from build123d import *

# Parameters (mm, degrees)
SKETCH_1_W          = 22
SKETCH_1_H          = 22
EXTRUDE_1_DEPTH     = 12
SKETCH_3_R          = 3.5
CUT_EXTRUDE_2_DEPTH = 12
SKETCH_5_R          = 1.5
EXTRUDE_2_DEPTH     = 4
SKETCH_6_W          = 12
SKETCH_6_H          = 22
EXTRUDE_3_DEPTH     = 22
SKETCH_7_R          = 4
CUT_EXTRUDE_3_DEPTH = 22


with BuildPart() as part:
    # 草图1 → 凸台-拉伸1 (new body)
    with BuildSketch(Plane.XY):
        Rectangle(SKETCH_1_W, SKETCH_1_H)
    extrude(amount=EXTRUDE_1_DEPTH)

    # 草图3 → 切除-拉伸2 (cut)
    with BuildSketch(Plane.XY.offset(12)):
        Circle(SKETCH_3_R)
    extrude(amount=-CUT_EXTRUDE_2_DEPTH, mode=Mode.SUBTRACT)

    # 草图5 → 凸台-拉伸2 (add)
    with BuildSketch(Plane(origin=(0, 0, 0), x_dir=(-1, 0, 0), z_dir=(0, 0, -1))):
        with Locations(Location((0, 8, 0), (0, 0, 180))):
            Circle(SKETCH_5_R)
        with Locations(Location((8, 0, 0), (0, 0, 180))):
            Circle(SKETCH_5_R)
        with Locations(Location((0, -8, 0), (0, 0, 180))):
            Circle(SKETCH_5_R)
        with Locations(Location((-8, 0, 0), (0, 0, 180))):
            Circle(SKETCH_5_R)
    extrude(amount=EXTRUDE_2_DEPTH)

    # 草图6 → 凸台-拉伸3 (add)
    with BuildSketch(Plane.ZY.offset(11)):
        with Locations((6, 0)):
            Rectangle(SKETCH_6_W, SKETCH_6_H)
    extrude(amount=EXTRUDE_3_DEPTH)

    # 草图7 → 切除-拉伸3 (cut)
    with BuildSketch(Plane.XZ.offset(11)):
        with Locations(Location((-26, 6, 0), (0, 0, 270))):
            Circle(SKETCH_7_R)
    extrude(amount=-CUT_EXTRUDE_3_DEPTH, mode=Mode.SUBTRACT)


solid = part.part
Part model, mm, in its own coordinate system. A direction names the side the tool comes from. Give positions to 0.01 mm unless a question says otherwise; leave off trailing zeros. Loops run counter-clockwise (first coordinate to the right, second up) from the corner with the lowest first, then second, coordinate; pieces in that order, holes last. Notation, with made-up numbers: M 25.25,1 L 32.25,1 A20 cw 32.25,33 Z; hole C 1,66 d10. An arc over 180 degrees is marked long. Put each result on its own line as item: value. Start each with the question number.
1) Flat gauge pins, fed straight in: pin 1 (4 mm diameter, centred on x = 5.5, y = -8, fed in from -Z); pin 2 (1.5 mm diameter, centred on x = -26, z = 3.5, fed in from +Y); pin 3 (8 mm diameter, centred on x = -23.5, z = 7.5, fed in from -Y). Where does each tip first touch, or does it go through?
2) Saw through at B-B (x = -26). List the corners of the cut face in (y, z).
3) Pull direction Y, two halves, no side cores. Call faces 3 (the cylindrical face through (-0.325, 9.464, -1.972)), 4 (the flat face through (-11, -11, 6)), 5 (the flat face through (-33, 0, 6)), 6 (the cylindrical face through (-9.5, -0.07, -1.97)): +Y half, -Y half, draft (parallel to the pull), parting line (faces both ways), or undercut.
4) Saw through at C-C (z = 5.5). List the corners of the cut face in (x, y).
5) 3-axis set-ups, long thin cutter, end or side, ignore diameter. For faces 1 (the flat face through (8, 0, -4)), 2 (the cylindrical face through (-0.325, -6.536, -1.972)): which of +Z, -Z, +X, -X, +Y, -Y reach the whole face in a straight line?
6) Saw through at A-A (y = 0). List the corners of the cut face in (x, z).
7) Saw through at D-D (x = 8). List the corners of the cut face in (y, z), then the cut area to 3 significant figures.
8) Probe probe 1 along X at (y, z) = (2.5, 6); probe 2 along Y at (x, z) = (0, 3.75); probe 3 along X at (y, z) = (-7.25, 6). List the from-to ranges inside material, lowest first.
Numbers:
1. pin 1: z = 0
1. pin 2: through
1. pin 3: y = -11
2. outline: M -11,0 L 11,0 L 11,2 L -11,2 Z; M -11,10 L 11,10 L 11,12 L -11,12 Z
3. face 3: undercut
3. face 4: -Y half
3. face 5: draft
3. face 6: parting line
4. outline: M -33,-11 L -29.97,-11 L -29.97,11 L -33,11 Z; M -22.03,-11 L 11,-11 L 11,11 L -22.03,11 Z; hole C 0,0 d7
5. face 1: -Z, +X, -X, +Y, -Y
5. face 2: -Z
6. outline: M -33,0 L -9.5,0 L -9.5,-4 L -6.5,-4 L -6.5,0 L -3.5,0 L -3.5,12 L -33,12 Z; M 3.5,0 L 6.5,0 L 6.5,-4 L 9.5,-4 L 9.5,0 L 11,0 L 11,12 L 3.5,12 Z; hole C -26,6 d8
7. outline: M -11,0 L -1.5,0 L -1.5,-4 L 1.5,-4 L 1.5,0 L 11,0 L 11,12 L -11,12 Z
7. area: 276 mm^2
8. probe 1: -33 to -30, -22 to -2.45, 2.45 to 11
8. probe 2: -11 to -3.5, 3.5 to 11
8. probe 3: -33 to -30, -22 to 11
